Read the model definition and answer for the solid it produces. Units are mm, in the model's axes. Face numbers are marked on the shaded views. A direction names the side the tool comes from. Coordinates: 2 decimals unless noted, no trailing zeros. Loops run counter-clockwise (first coordinate to the right, second up) from the corner with the lowest first, then second, coordinate; pieces in that order, holes last.
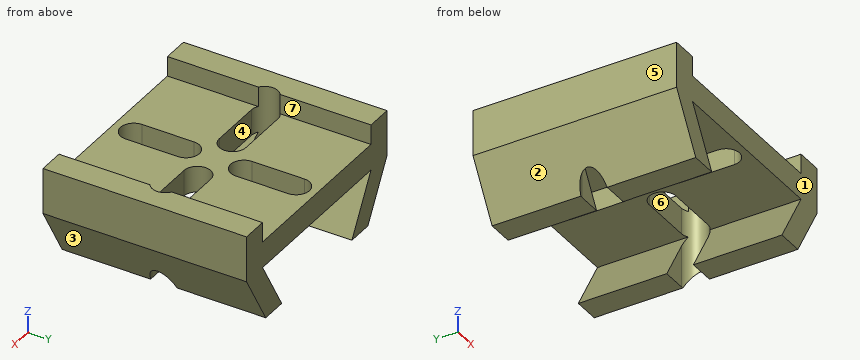
from build123d import *

# Parameters (mm, degrees)
EXTRUDE_1_DEPTH     = 39
CUT_EXTRUDE_1_DEPTH = 49.716984362


with BuildPart() as part:
    # 草图1 → 凸台-拉伸1 (new body)
    with BuildSketch(Plane(origin=(0, 0, 0), x_dir=(1, 0, 0), z_dir=(0, 1, 0))):
        Polygon((-22, 0), (-22, -3.8), (-17, -3.8), (-17, 0), (17, 0), (17, -3.8), (22, -3.8), (22, 0), (22, 5), (16, 15.392304845), (11, 15.392304845), (17, 5), (-17, 5), (-11, 15.392304845), (-16, 15.392304845), (-22, 5), align=None)
    extrude(amount=EXTRUDE_1_DEPTH)

    # 草图2 → 切除-拉伸1 (cut, through all)
    with BuildSketch(Plane.XY.offset(3.8)):
        with BuildLine():
            Line((-2.548549229, 25.043167775), (-2.548549229, 35.043167775))
            ThreePointArc((-2.548549229, 35.043167775), (0, 37.591717003), (2.548549229, 35.043167775))
            Line((2.548549229, 35.043167775), (2.548549229, 25.043167775))
            ThreePointArc((2.548549229, 25.043167775), (0, 22.494618546), (-2.548549229, 25.043167775))
        make_face()
        with BuildLine():
            Line((5.543167775, 16.951450771), (15.543167775, 16.951450771))
            ThreePointArc((15.543167775, 16.951450771), (18.091717003, 19.5), (15.543167775, 22.048549229))
            Line((15.543167775, 22.048549229), (5.543167775, 22.048549229))
            ThreePointArc((5.543167775, 22.048549229), (2.994618546, 19.5), (5.543167775, 16.951450771))
        make_face()
        with BuildLine():
            Line((-2.548549229, 13.956832225), (-2.548549229, 3.956832225))
            ThreePointArc((-2.548549229, 3.956832225), (0, 1.408282997), (2.548549229, 3.956832225))
            Line((2.548549229, 3.956832225), (2.548549229, 13.956832225))
            ThreePointArc((2.548549229, 13.956832225), (0, 16.505381454), (-2.548549229, 13.956832225))
        make_face()
        with BuildLine():
            Line((-5.543167775, 22.048549229), (-15.543167775, 22.048549229))
            ThreePointArc((-15.543167775, 22.048549229), (-18.091717003, 19.5), (-15.543167775, 16.951450771))
            Line((-15.543167775, 16.951450771), (-5.543167775, 16.951450771))
            ThreePointArc((-5.543167775, 16.951450771), (-2.994618546, 19.5), (-5.543167775, 22.048549229))
        make_face()
    extrude(amount=-CUT_EXTRUDE_1_DEPTH, mode=Mode.SUBTRACT)


solid = part.part
Q1. A cutting plane is placed at A-A (x = 0). Give the vertices of the cut face in (y, z).
Findings below:
outline: (0, -5) - (1.41, -5) - (1.41, 0) - (0, 0) - close; (16.51, -5) - (22.49, -5) - (22.49, 0) - (16.51, 0) - close; (37.59, -5) - (39, -5) - (39, 0) - (37.59, 0) - close
Q2. A cutting plane is placed at B-B (y = 4.5). Give the vertices of the cut face in (x, z).
Findings below:
outline: (-22, -5) - (-16, -15.39) - (-11, -15.39) - (-17, -5) - (-2.55, -5) - (-2.55, 0) - (-17, 0) - (-17, 3.8) - (-22, 3.8) - close; (2.55, -5) - (17, -5) - (11, -15.39) - (16, -15.39) - (22, -5) - (22, 3.8) - (17, 3.8) - (17, 0) - (2.55, 0) - close
Q3. Which of the six approach directions +Z, -Z, +X, -X, +Y, -Y give full straight-line access (tool end or side, diameter ignored) to the marked faces 5, 6 and 7?
Findings below:
face 5: +Z, -Z, -X, +Y, -Y
face 6: +Z, -Z
face 7: +Z, +Y, -Y
Q4. A cutting plane is placed at D-D (z = -9). Give the vertices of the cut face in (x, y), then the cut area to 3 significant figures.
Findings below:
outline: (-19.69, 0) - (-14.69, 0) - (-14.69, 16.95) - (-15.54, 16.95) arc R2.55 cw to (-15.54, 22.05) - (-14.69, 22.05) - (-14.69, 39) - (-19.69, 39) - close; (14.69, 0) - (19.69, 0) - (19.69, 39) - (14.69, 39) - (14.69, 22.05) - (15.54, 22.05) arc R2.55 cw to (15.54, 16.95) - (14.69, 16.95) - close
area: 361 mm2
Q5. Straight lines are drawn through the part: probe 1 along Y at (x, z) = (15, -14.5); probe 2 along Z at (x, y) = (-10.5, 13); probe 3 along X at (y, z) = (10.5, -11.5). For each, find the intervals that lie inside material, in ascending order.
Findings below:
probe 1: y = 0 to 16.95, 22.05 to 39
probe 2: z = -5 to 0
probe 3: x = -18.25 to -13.25, 13.25 to 18.25
Q6. Flat-ended cylindrical pins translate along their axes: pin 1 Ø8 at (x, z) = (-16.5, -5.5) entering from -Y; pin 2 Ø3 at (x, z) = (-12, -8) entering from +Y; pin 3 Ø8 at (x, y) = (-0.5, 13) entering from -Z; pin 4 Ø6 at (y, z) = (16, -13) entering from +X. Find the tip coordinate at first contact, or state that the pin passes through.
Findings below:
pin 1: stops at y = 0
pin 2: passes through
pin 3: stops at z = -5
pin 4: stops at x = 19.11
Q7. Determine the mould class of the marked faces 1, 2, 3 and 4 for opening direction X: +X half, -X half, draft (parallel to the pull), parting line (faces both ways), or undercut.
Findings below:
face 1: draft
face 2: -X half
face 3: +X half
face 4: undercut
Q8. A cutting plane is placed at C-C (z = -3.5). Give the vertices of the cut face in (x, y).
Findings below:
outline: (-22, 0) - (22, 0) - (22, 39) - (-22, 39) - close; hole (-15.54, 16.95) - (-5.54, 16.95) arc R2.55 ccw to (-5.54, 22.05) - (-15.54, 22.05) arc R2.55 ccw to start; hole (-2.55, 3.96) arc R2.55 ccw to (2.55, 3.96) - (2.55, 13.96) arc R2.55 ccw to (-2.55, 13.96) - close; hole (-2.55, 25.04) arc R2.55 ccw to (2.55, 25.04) - (2.55, 35.04) arc R2.55 ccw to (-2.55, 35.04) - close; hole (5.54, 16.95) - (15.54, 16.95) arc R2.55 ccw to (15.54, 22.05) - (5.54, 22.05) arc R2.55 ccw to start
